```python
from build123d import *

# Parameters (mm, degrees)
RESSALTO_EXTRUS_O1_DEPTH = 50
RESSALTO_EXTRUS_O2_DEPTH = 10
RESSALTO_EXTRUS_O3_START = 10
RESSALTO_EXTRUS_O3_DEPTH = 10
ESBO_O4_R                = 11
RESSALTO_EXTRUS_O4_DEPTH = 15
RESSALTO_EXTRUS_O5_START = 15
ESBO_O5_R                = 11
RESSALTO_EXTRUS_O5_DEPTH = 15
ESBO_O6_R                = 7.5
CORTE_EXTRUS_O1_DEPTH    = 200
ESBO_O7_R                = 11
RESSALTO_EXTRUS_O6_DEPTH = 15
ESBO_O8_R                = 7.5
CORTE_EXTRUS_O2_DEPTH    = 30


with BuildPart() as part:
    # Esboço1 → Ressalto-extrusão1 (new body)
    with BuildSketch(Plane(origin=(0, 0, 0), x_dir=(1, 0, 0), z_dir=(0, 1, 0))):
        with BuildLine():
            Line((40, 60), (-40, 60))
            ThreePointArc((-40, 60), (-54.142135624, 54.142135624), (-60, 40))
            Line((-60, 40), (-60, -40))
            ThreePointArc((-60, -40), (-54.142135624, -54.142135624), (-40, -60))
            Line((-40, -60), (40, -60))
            ThreePointArc((40, -60), (54.142135624, -54.142135624), (60, -40))
            Line((60, -40), (60, 40))
            ThreePointArc((60, 40), (54.142135624, 54.142135624), (40, 60))
        make_face()
        with BuildLine():
            Line((40, -50), (-40, -50))
            ThreePointArc((-40, -50), (-47.071067812, -47.071067812), (-50, -40))
            Line((-50, -40), (-50, 40))
            ThreePointArc((-50, 40), (-47.071067812, 47.071067812), (-40, 50))
            Line((-40, 50), (40, 50))
            ThreePointArc((40, 50), (47.071067812, 47.071067812), (50, 40))
            Line((50, 40), (50, -40))
            ThreePointArc((50, -40), (47.071067812, -47.071067812), (40, -50))
        make_face(mode=Mode.SUBTRACT)
    extrude(amount=RESSALTO_EXTRUS_O1_DEPTH)

    # Esboço2 → Ressalto-extrusão2 (add)
    with BuildSketch(Plane(origin=(0, 50, 0), x_dir=(1, 0, 0), z_dir=(0, 1, 0))):
        with BuildLine():
            Line((-40, -60), (40, -60))
            ThreePointArc((40, -60), (54.142135624, -54.142135624), (60, -40))
            Line((60, -40), (60, 40))
            ThreePointArc((60, 40), (54.142135624, 54.142135624), (40, 60))
            Line((40, 60), (-40, 60))
            ThreePointArc((-40, 60), (-54.142135624, 54.142135624), (-60, 40))
            Line((-60, 40), (-60, -40))
            ThreePointArc((-60, -40), (-54.142135624, -54.142135624), (-40, -60))
        make_face()
    extrude(amount=RESSALTO_EXTRUS_O2_DEPTH)

    # Esboço3 → Ressalto-extrusão3 (add)
    with BuildSketch(Plane(origin=(0, 0, 0), x_dir=(-1, 0, 0), z_dir=(0, -1, 0)).offset(RESSALTO_EXTRUS_O3_START)):
        with BuildLine():
            Line((40, -60), (-40, -60))
            ThreePointArc((-40, -60), (-54.142135624, -54.142135624), (-60, -40))
            Line((-60, -40), (-60, 40))
            ThreePointArc((-60, 40), (-54.142135624, 54.142135624), (-40, 60))
            Line((-40, 60), (40, 60))
            ThreePointArc((40, 60), (54.142135624, 54.142135624), (60, 40))
            Line((60, 40), (60, -40))
            ThreePointArc((60, -40), (54.142135624, -54.142135624), (40, -60))
        make_face()
    extrude(amount=-RESSALTO_EXTRUS_O3_DEPTH)

    # Esboço4 → Ressalto-extrusão4 (add)
    with BuildSketch(Plane.ZY.offset(60)):
        with Locations(Location((20, 25, 0), (0, 0, 180))):
            Circle(ESBO_O4_R)
        with Locations(Location((-20, 25, 0), (0, 0, 180))):
            Circle(ESBO_O4_R)
    extrude(amount=RESSALTO_EXTRUS_O4_DEPTH)

    # Esboço5 → Ressalto-extrusão5 (add)
    with BuildSketch(Plane(origin=(60, 0, 0), x_dir=(0, 0, -1), z_dir=(1, 0, 0)).offset(RESSALTO_EXTRUS_O5_START)):
        with Locations((-20, 25)):
            Circle(ESBO_O5_R)
        with Locations((20, 25)):
            Circle(ESBO_O5_R)
    extrude(amount=-RESSALTO_EXTRUS_O5_DEPTH)

    # Esboço6 → Corte-extrusão1 (cut)
    with BuildSketch(Plane.ZY.offset(75)):
        with Locations((20, 25)):
            Circle(ESBO_O6_R)
        with Locations((-20, 25)):
            Circle(ESBO_O6_R)
    extrude(amount=-CORTE_EXTRUS_O1_DEPTH, mode=Mode.SUBTRACT)

    # Esboço7 → Ressalto-extrusão6 (add)
    with BuildSketch(Plane(origin=(0, 60, 0), x_dir=(1, 0, 0), z_dir=(0, 1, 0))):
        with Locations(Location((0, 0, 0), (0, 0, 270))):
            Circle(ESBO_O7_R)
    extrude(amount=RESSALTO_EXTRUS_O6_DEPTH)

    # Esboço8 → Corte-extrusão2 (cut)
    with BuildSketch(Plane(origin=(0, 75, 0), x_dir=(1, 0, 0), z_dir=(0, 1, 0))):
        with Locations(Location((0, 0, 0), (0, 0, 270))):
            Circle(ESBO_O8_R)
    extrude(amount=-CORTE_EXTRUS_O2_DEPTH, mode=Mode.SUBTRACT)


solid = part.part
```
Input: part model. Units: mm. Frame: model coordinates. A direction names the side the tool comes from. Coordinates: 2 decimals unless noted, no trailing zeros. Loops run counter-clockwise (first coordinate to the right, second up) from the corner with the lowest first, then second, coordinate; pieces in that order, holes last. Notation, with made-up numbers: M -12.75,71 L 14.25,71 A27 ccw 14.25,106 Z; hole C 79.25,2.25 d9. An arc over 180 degrees is marked long. Use a Markdown table: item, result. Add a question column.
1) Pin query (flat end, axial travel): P1, Ø2, axis at x = -21, z = -13.5, coming from the +Y side. Return the tip coordinate at first contact, or that it passes through.
2) Set-up query: faces 1 (the flat face through (2.6, 75, 7.2)), 2 (the cylindrical face through (-10.74, 67.4, -2.38)), 3 (the cylindrical face through (67.605, 15.241, -25.076)), 4 (the cylindrical face through (46.99, 24.65, -47.15)). Return all of +Z, -Z, +X, -X, +Y, -Y with unobstructed straight access to the full face (end or side cutting, diameter ignored); none if empty.
3) Section B-B, the plane z = 35.5. Return the cut outline in (x, y), plus the area to 3 significant figures.
4) Line query: L1, parallel to Z at x = 11.5, y = 15.5; L2, parallel to Y at x = 61, z = -20; L3, parallel to Y at x = -55, z = -20. Output: solid intervals per line, ascending. Write a range as from..to.
5) Section A-A, the plane z = -20. Return the cut outline in (x, y), plus the area to 3 significant figures.
6) Draft query along Y for faces 5 (the flat face through (1, 25, 50)), 6 (the cylindrical face through (-67.395, 34.759, 14.924)), 7 (the cylindrical face through (54.297, 24.51, -53.986)). Return one class per face: +Y half, -Y half, draft (parallel to the pull), parting line (faces both ways), or undercut.
7) Section C-C, the plane x = 0. Return the cut outline in (y, z).
8) Section D-D, the plane y = 4.5. Return the cut outline in (x, z), plus the area to 3 significant figures.
Answer below:
| question | item | result |
|---|---|---|
| 1 | P1 | y = 60 |
| 2 | face 1 | +Z, -Z, +X, -X, +Y |
| 2 | face 2 | +Y |
| 2 | face 3 | +X |
| 2 | face 4 | none |
| 3 | outline | M -60,-10 L 60,-10 L 60,60 L -60,60 Z; hole M -50,0 L 50,0 L 50,50 L -50,50 Z |
| 3 | area | 3,400 mm2 |
| 4 | L1 | -60..-50, 50..60 |
| 4 | L2 | 14..17.5, 32.5..36 |
| 4 | L3 | -10..17.5, 32.5..60 |
| 5 | outline | M -75,14 L -60,14 L -60,-10 L 60,-10 L 60,14 L 75,14 L 75,17.5 L 50,17.5 L 50,0 L -50,0 L -50,17.5 L -75,17.5 Z; M -75,32.5 L -50,32.5 L -50,50 L 50,50 L 50,32.5 L 75,32.5 L 75,36 L 60,36 L 60,60 L -60,60 L -60,36 L -75,36 Z |
| 5 | area | 3,310 mm2 |
| 6 | face 5 | undercut |
| 6 | face 6 | parting line |
| 6 | face 7 | draft |
| 7 | outline | M -10,-60 L 60,-60 L 60,-11 L 75,-11 L 75,-7.5 L 50,-7.5 L 50,-50 L 0,-50 L 0,50 L 50,50 L 50,7.5 L 75,7.5 L 75,11 L 60,11 L 60,60 L -10,60 Z |
| 8 | outline | M -60,-40 A20 ccw -40,-60 L 40,-60 A20 ccw 60,-40 L 60,40 A20 ccw 40,60 L -40,60 A20 ccw -60,40 Z; hole M -50,-40 A10 ccw -40,-50 L 40,-50 A10 ccw 50,-40 L 50,40 A10 ccw 40,50 L -40,50 A10 ccw -50,40 Z |
| 8 | area | 4,140 mm2 |
